Work out the finished part from the listing and answer in its coordinate system (mm). Round coordinates to 2 decimals unless told otherwise and drop trailing zeros. Write each loop counter-clockwise with the first axis right and the second up, starting at its lowest first coordinate (ties: lowest second). Pieces come first, ordered by that corner, then holes. Notation, with made-up numbers: (-36, 19.25) - (9, 19.25) arc R21 cw to (9, 44.25) - close; hole circle Ø5 at (-32, 75). An arc over 180 degrees is marked (long way). Answer as a JSON object with one key per item and string values.
```python
from build123d import *

# Parameters (mm, degrees)
SKETCH1_R           = 6.736700536
BOSS_EXTRUDE1_DEPTH = 3
FILLET1_R           = 5
FILLET2_R           = 5


with BuildPart() as part:
    # Sketch1 → Boss-Extrude1 (new body)
    with BuildSketch(Plane(origin=(0, 0, 0), x_dir=(1, 0, 0), z_dir=(0, 1, 0))):
        Polygon((-51.5, -13), (-51.5, -53), (-8.5, -53), (-8.5, -50), (11.5, -50), (11.5, -53), (51.5, -53), (51.5, -10), (48.5, -10), (48.5, 10), (51.5, 10), (51.5, 50), (8.5, 50), (8.5, 47), (-11.5, 47), (-11.5, 50), (-51.5, 50), (-51.5, 7), (-48.5, 7), (-48.5, -13), align=None)
        Polygon((-40.119028072, -29.730929333), (-40.119028072, 29.730929333), (-10.573569788, 0), align=None, mode=Mode.SUBTRACT)
        Polygon((-29.545458284, 37.370874503), (29.545458284, 37.370874503), (4.043573282, 11.708901907), (-0.025303783, 7.665407798), align=None, mode=Mode.SUBTRACT)
        Polygon((40.119028072, 29.730929333), (40.119028072, -29.730929333), (10.573569788, 0), align=None, mode=Mode.SUBTRACT)
        Polygon((29.545458284, -40.370874503), (-29.545458284, -40.370874503), (0, -10.63994517), align=None, mode=Mode.SUBTRACT)
        with Locations(Location((0, 0, 0), (0, 0, 270))):
            Circle(SKETCH1_R, mode=Mode.SUBTRACT)
    extrude(amount=BOSS_EXTRUDE1_DEPTH)

    # Fillet1
    fillet1_edges = [part.edges().sort_by_distance(p)[0] for p in [
        (29.545458284, 1.5, 40.370874503),
        (-29.545458284, 1.5, 40.370874503),
        (-40.119028072, 1.5, -29.730929333),
        (-40.119028072, 1.5, 29.730929333),
        (29.545458284, 1.5, -37.370874503),
        (-29.545458284, 1.5, -37.370874503),
        (40.119028072, 1.5, 29.730929333),
        (40.119028072, 1.5, -29.730929333),
    ]]
    fillet(fillet1_edges, radius=FILLET1_R)

    # Fillet2
    fillet2_edges = [part.edges().sort_by_distance(p)[0] for p in [
        (0, 1.5, 10.63994517),
        (-10.573569788, 1.5, 0),
        (-0.025303783, 1.5, -7.665407798),
        (10.573569788, 1.5, 0),
    ]]
    fillet(fillet2_edges, radius=FILLET2_R)


solid = part.part
```
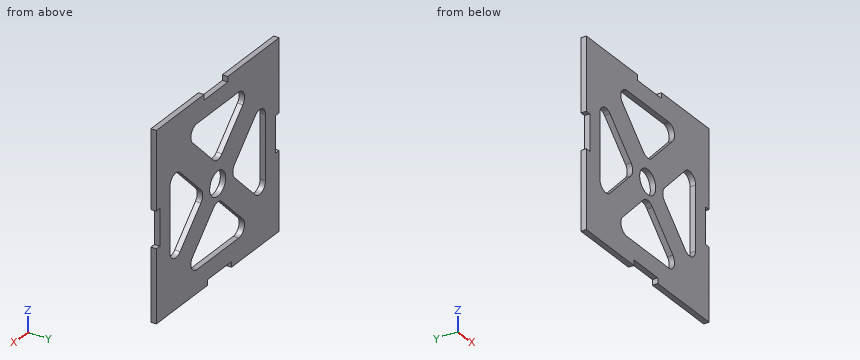
Item 1: A cutting plane is placed at A-A (x = 0). Write down the section's boundary in (y, z), and give its area (3 significant figures).
Results found:
{"outline": "(0, -47) - (3, -47) - (3, -37.37) - (0, -37.37) - close; (0, -9.74) - (3, -9.74) - (3, -6.74) - (0, -6.74) - close; (0, 6.74) - (3, 6.74) - (3, 12.73) - (0, 12.73) - close; (0, 40.37) - (3, 40.37) - (3, 50) - (0, 50) - close", "area": "84.8 mm²"}
Item 2: Consider line 1 along X through (y, z) = (0.7, 0); line 2 along Z through (x, y) = (36, 2.1); line 3 along Z through (x, y) = (-10, 1.4). Determine where each line is inside the solid, lowest interval first.
Results found:
{"line 1": "-48.5 to -40.12, -12.62 to -6.74, 6.74 to 12.62, 40.12 to 48.5", "line 2": "-50 to -22.53, 22.53 to 53", "line 3": "-47 to -37.37, -17.7 to 20.7, 40.37 to 53"}
Item 3: A cutting plane is placed at C-C (z = -24). Write down the section's boundary in (x, y).
Results found:
{"outline": "(-51.5, 0) - (-16.26, 0) - (-16.26, 3) - (-51.5, 3) - close; (16.26, 0) - (51.5, 0) - (51.5, 3) - (16.26, 3) - close"}
Item 4: Each of these flat-tipped pins is pushed along its axis until it touches: P1, Ø12, axis at x = -2, z = -17, coming from the -Y side; P2, Ø11, axis at x = 0, z = 0, coming from the +Y side; P3, Ø1.5, axis at x = -2.5, y = 2, coming from the +Z side. Where does it stop, or does it pass through?
Results found:
{"P1": "y = 0", "P2": "through", "P3": "z = 50"}
Item 5: A cutting plane is placed at D-D (x = 24). Write down the section's boundary in (y, z), and give its area (3 significant figures).
Results found:
{"outline": "(0, -50) - (3, -50) - (3, -13.51) - (0, -13.51) - close; (0, 13.51) - (3, 13.51) - (3, 53) - (0, 53) - close", "area": "228 mm²"}
Item 6: A cutting plane is placed at B-B (z = 0). Write down the section's boundary in (x, y).
Results found:
{"outline": "(-48.5, 0) - (-40.12, 0) - (-40.12, 3) - (-48.5, 3) - close; (-12.62, 0) - (-6.74, 0) - (-6.74, 3) - (-12.62, 3) - close; (6.74, 0) - (12.62, 0) - (12.62, 3) - (6.74, 3) - close; (40.12, 0) - (48.5, 0) - (48.5, 3) - (40.12, 3) - close"}
